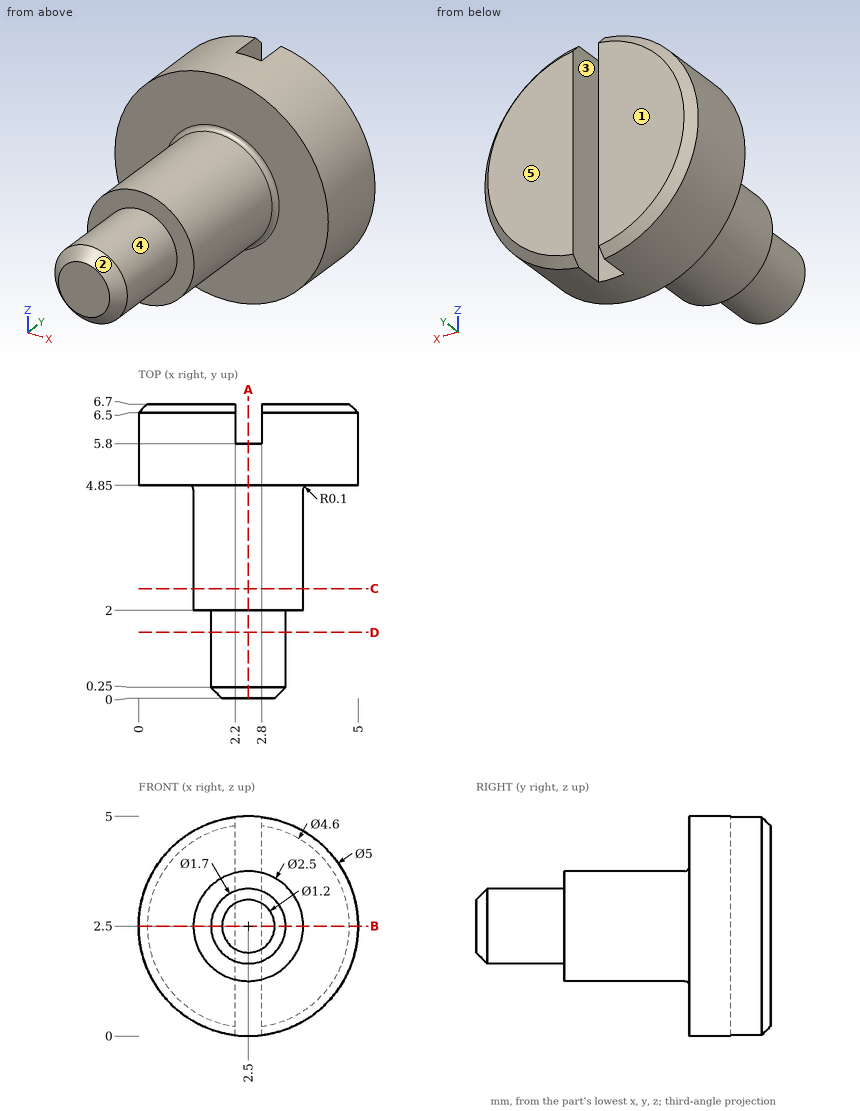
Geometry: see drawing. Coordinates: mm, zero at the bounding-box minimum. A direction names the side the tool comes from. Give positions to 0.01 mm unless a question says otherwise; leave off trailing zeros. Order: outer loops, then holes, each group sorted by start corner. A loop starts at its lowest first (then second) coordinate and runs counter-clockwise, first axis right, second up. Notation, with made-up numbers: M -32.75,66 L -2.75,66 A20 cw -2.75,95 Z; hole C 23.25,13 d2. An arc over 180 degrees is marked long. Answer as CSV lines item,"result". Start each with the question number.
1) Cut plane D-D (y = 1.5). Output: boundary loops of the cut face in (x, z), then the cut area to 3 significant figures.
2) Set-up query: the marked faces 4 and 5. Return all of +Z, -Z, +X, -X, +Y, -Y with unobstructed straight access to the full face (end or side cutting, diameter ignored); none if empty.
3) Cut plane A-A (x = 2.5). Output: boundary loops of the cut face in (y, z).
4) Line query: line 1 (X direction, y = 6, z = 2); line 2 (Y direction, x = 1.8, z = 1.3); line 3 (X direction, y = 6, z = 0.45). Output: solid intervals per line, ascending. Write a range as from..to.
5) Mould query, pull axis X, two halves, no side actions, for the marked faces 1, 2 and 3. Classes: +X half, -X half, draft (parallel to the pull), parting line (faces both ways), or undercut.
6) Cut plane C-C (y = 2.5). Output: boundary loops of the cut face in (x, z).
7) Cut plane B-B (z = 2.5). Output: boundary loops of the cut face in (x, y), then the cut area to 3 significant figures.
8) First-contact query: P1, Ø1, axis at x = 3.5, y = 3.5, coming from the -Z side; P2, Ø1, axis at y = 1, z = 1.5, coming from the +X side; P3, Ø1, axis at x = 4, y = 2.5, coming from the -Z side. Flat tips, straight axial feed; report the tip coordinate or a pass-through.
Findings below:
1,outline,"C 2.5,2.5 d1.7"
1,area,"2.27 mm²"
2,face 4,"-Y"
2,face 5,"+Z, -Z, +X, -X, +Y"
3,outline,"M 0,1.9 L 0.25,1.65 L 2,1.65 L 2,1.25 L 4.75,1.25 A0.1 cw 4.85,1.15 L 4.85,0 L 5.8,0 L 5.8,5 L 4.85,5 L 4.85,3.85 A0.1 cw 4.75,3.75 L 2,3.75 L 2,3.35 L 0.25,3.35 L 0,3.1 Z"
4,line 1,"x = 0.05..2.2, 2.8..4.95"
4,line 2,"y = 4.85..6.7"
4,line 3,"x = 1.07..2.2, 2.8..3.93"
5,face 1,"draft"
5,face 2,"parting line"
5,face 3,"undercut"
6,outline,"C 2.5,2.5 d2.5"
7,outline,"M 0,4.85 L 1.15,4.85 A0.1 cw 1.25,4.75 L 1.25,2 L 1.65,2 L 1.65,0.25 L 1.9,0 L 3.1,0 L 3.35,0.25 L 3.35,2 L 3.75,2 L 3.75,4.75 A0.1 cw 3.85,4.85 L 5,4.85 L 5,6.5 L 4.8,6.7 L 2.8,6.7 L 2.8,5.8 L 2.2,5.8 L 2.2,6.7 L 0.2,6.7 L 0,6.5 Z"
7,area,"19.1 mm²"
8,P1,"stops at z = 1.35"
8,P2,"stops at x = 3.19"
8,P3,"stops at z = 1.75"
